```python
from build123d import *

# Parameters (mm, degrees)
BOARD_DEPTH = 1.6194


with BuildPart() as part:
    # Sketch1 → Board (new body)
    with BuildSketch(Plane.XY):
        with BuildLine():
            Line((10, 29), (10, 57.01299))
            ThreePointArc((10, 57.01299), (10.185190901, 57.290158106), (10.51213, 57.22513))
            ThreePointArc((10.51213, 57.22513), (12.777621512, 57.222368475), (12.77487, 59.48786))
            ThreePointArc((12.77487, 59.48786), (12.709829188, 59.814802566), (12.987, 60))
            Line((12.987, 60), (21.95, 60))
            ThreePointArc((21.95, 60), (22.657106781, 59.707106781), (22.95, 59))
            Line((22.95, 59), (22.95, 53))
            ThreePointArc((22.95, 53), (23.242893219, 52.292893219), (23.95, 52))
            Line((23.95, 52), (32.05, 52))
            ThreePointArc((32.05, 52), (32.757106781, 52.292893219), (33.05, 53))
            Line((33.05, 53), (33.05, 59))
            ThreePointArc((33.05, 59), (33.342893219, 59.707106781), (34.05, 60))
            Line((34.05, 60), (37.01299, 60))
            ThreePointArc((37.01299, 60), (37.290150019, 59.814804479), (37.22512, 59.48787))
            ThreePointArc((37.22512, 59.48787), (37.223732391, 57.223742391), (39.48786, 57.22513))
            ThreePointArc((39.48786, 57.22513), (39.814807186, 57.290168899), (40, 57.01299))
            Line((40, 57.01299), (40, 29))
            ThreePointArc((40, 29), (39.121323273, 26.878676727), (37, 26))
            Line((37, 26), (13, 26))
            ThreePointArc((13, 26), (10.878679656, 26.878679656), (10, 29))
        make_face()
    extrude(amount=BOARD_DEPTH)


solid = part.part
```
Read the model definition and answer for the solid it produces. Units are mm, in the model's axes. A direction names the side the tool comes from. Round coordinates to 2 decimals unless told otherwise and drop trailing zeros. Write each loop counter-clockwise with the first axis right and the second up, starting at its lowest first coordinate (ties: lowest second). Pieces come first, ordered by that corner, then holes. Notation, with made-up numbers: (-37.75, 84) - (-13.75, 84) arc R22 ccw to (-13.75, 90) - close; hole circle Ø2 at (-12, 89.25). An arc over 180 degrees is marked (long way). One line per item, written item: value.
Q1. Find section B-B (x = 30.5). Determine the outline of the cut face in (y, z), and give its area (3 significant figures).
The answers:
outline: (26, 0) - (52, 0) - (52, 1.62) - (26, 1.62) - close
area: 42.1 mm2
Q2. Which of the six approach directions +Z, -Z, +X, -X, +Y, -Y give full straight-line access (tool end or side, diameter ignored) to faces 1 (the flat face through (28, 52, 1)), 2 (the flat face through (10, 43, 1))?
The answers:
face 1: +Z, -Z, +Y
face 2: +Z, -Z, -X, +Y, -Y
Q3. Find section C-C (z = 0.5). Determine the outline of the cut face in (x, y).
The answers:
outline: (10, 29) arc R3 ccw to (13, 26) - (37, 26) arc R3 ccw to (40, 29) - (40, 57.01) arc R0.3 ccw to (39.49, 57.23) arc R1.6 cw to (37.23, 59.49) arc R0.3 ccw to (37.01, 60) - (34.05, 60) arc R1 ccw to (33.05, 59) - (33.05, 53) arc R1 cw to (32.05, 52) - (23.95, 52) arc R1 cw to (22.95, 53) - (22.95, 59) arc R1 ccw to (21.95, 60) - (12.99, 60) arc R0.3 ccw to (12.77, 59.49) arc R1.6 cw to (10.51, 57.23) arc R0.3 ccw to (10, 57.01) - close
Q4. Find section A-A (y = 54.5). Determine the outline of the cut face in (x, z), and give its area (3 significant figures).
The answers:
outline: (10, 0) - (22.95, 0) - (22.95, 1.62) - (10, 1.62) - close; (33.05, 0) - (40, 0) - (40, 1.62) - (33.05, 1.62) - close
area: 32.2 mm2
Q5. Straight lines are drawn through the part: line 1 (X direction, y = 56, z = 1.15); line 2 (Y direction, x = 26, z = 1.45); line 3 (X direction, y = 57, z = 0.45). For each, find the intervals that lie inside material, in ascending order. Write a range as from..to.
The answers:
line 1: x = 10..22.95, 33.05..40
line 2: y = 26..52
line 3: x = 10..10.79, 12.5..22.95, 33.05..37.5, 39.21..40
